Design review of the part built by this model. Coordinates are the model's own, in mm. A direction names the side the tool comes from. Coordinates: 2 decimals unless noted, no trailing zeros. Order: outer loops, then holes, each group sorted by start corner. A loop starts at its lowest first (then second) coordinate and runs counter-clockwise, first axis right, second up. Notation, with made-up numbers: M -6.75,2 L 52.25,2 A22 cw 52.25,37 Z; hole C -22,-11 d2. An arc over 180 degrees is marked long. Answer in a Markdown table with one row per item.
from build123d import *

# Parameters (mm, degrees)
SCHIZZO1_R                           = 6.5
SCHIZZO1_R_2                         = 2
BASE_FLANGIA1_DEPTH                  = 4
PIEGATURA_START                      = -26
PIEGATURA_DELLO_SCHIZZO1_OUTLINE_W   = 50
PIEGATURA_DELLO_SCHIZZO1_OUTLINE_H   = 4
PIEGATURA_DELLO_SCHIZZO1_DEPTH       = 52
PIEGATURA_START_2                    = -30
PIEGATURA_DELLO_SCHIZZO1_2_OUTLINE_R = 6.5
PIEGATURA_DELLO_SCHIZZO1_2_DEPTH     = 4
PIEGATURA_DELLO_SCHIZZO1_3_DEPTH     = 52
PIEGATURA_START_3                    = -25
PIEGATURA_DELLO_SCHIZZO1_4_DEPTH     = 50
ESTRUSIONE_ESTRUSIONE1_DEPTH         = 2


with BuildPart() as part:
    # Base-Flangia1: sheet metal written as solids
    # Schizzo1 → Base-Flangia1 (new body)
    with BuildSketch(Plane.XY):
        with BuildLine():
            Line((-25, -72), (-25, 0))
            ThreePointArc((-25, 0), (0, 25), (25, 0))
            Line((25, 0), (25, -72))
            ThreePointArc((25, -72), (23.535533906, -75.535533906), (20, -77))
            Line((20, -77), (-20, -77))
            ThreePointArc((-20, -77), (-23.535533906, -75.535533906), (-25, -72))
        make_face()
        Circle(SCHIZZO1_R, mode=Mode.SUBTRACT)
        with Locations((-12.5, -67)):
            Circle(SCHIZZO1_R_2, mode=Mode.SUBTRACT)
        with Locations((12.5, -67)):
            Circle(SCHIZZO1_R_2, mode=Mode.SUBTRACT)
    extrude(amount=-BASE_FLANGIA1_DEPTH)

    # Piegatura dello schizzo1: read off the stored shape, not the designer's step
    # Piegatura dello schizzo1 outline → Piegatura dello schizzo1 (cut)
    with BuildSketch(Plane(origin=(0, 0, 0), x_dir=(1, 0, 0), z_dir=(0, 1, 0)).offset(PIEGATURA_START)):
        with Locations((0, 2)):
            Rectangle(PIEGATURA_DELLO_SCHIZZO1_OUTLINE_W, PIEGATURA_DELLO_SCHIZZO1_OUTLINE_H)
    extrude(amount=PIEGATURA_DELLO_SCHIZZO1_DEPTH, mode=Mode.SUBTRACT)

    # Piegatura dello schizzo1 2 outline → Piegatura dello schizzo1 2 (add)
    with BuildSketch(Plane(origin=(0, 0, 0), x_dir=(1, 0, 0), z_dir=(0, 1, 0)).offset(PIEGATURA_START_2)):
        with BuildLine():
            Line((-25, 0), (-25, -26.862699383))
            ThreePointArc((-25, -26.862699383), (0, -51.862699383), (25, -26.862699383))
            Line((25, -26.862699383), (25, 0))
            Line((25, 0), (-25, 0))
        make_face()
        with Locations((0, -26.862699383)):
            Circle(PIEGATURA_DELLO_SCHIZZO1_2_OUTLINE_R, mode=Mode.SUBTRACT)
    extrude(amount=PIEGATURA_DELLO_SCHIZZO1_2_DEPTH)

    # Piegatura dello schizzo1 3 outline → Piegatura dello schizzo1 3 (cut)
    with BuildSketch(Plane.YZ.offset(PIEGATURA_START)):
        with BuildLine():
            ThreePointArc((-26, 0.01), (-27.174501807, -2.825498193), (-30.01, -4))
            Line((-30.01, -4), (-26, -4))
            Line((-26, -4), (-26, 0.01))
        make_face()
    extrude(amount=PIEGATURA_DELLO_SCHIZZO1_3_DEPTH, mode=Mode.SUBTRACT)

    # Piegatura dello schizzo1 4 outline → Piegatura dello schizzo1 4 (add)
    with BuildSketch(Plane.YZ.offset(PIEGATURA_START_3)):
        with BuildLine():
            ThreePointArc((-30, 0.01), (-30.002928932, 0.002928932), (-30.01, 0))
            Line((-30.01, 0), (-30, 0))
            Line((-30, 0), (-30, 0.01))
        make_face()
    extrude(amount=PIEGATURA_DELLO_SCHIZZO1_4_DEPTH)

    # Schizzo13 → Estrusione-Estrusione1 (add)
    with BuildSketch(Plane.ZY.offset(25)):
        with BuildLine():
            Line((0.01, -30), (15, -30))
            Line((15, -30), (0, -45))
            Line((0, -45), (0, -30.01))
            ThreePointArc((0, -30.01), (0.002928932, -30.002928932), (0.01, -30))
        make_face()
    estrusione_estrusione1 = extrude(amount=-ESTRUSIONE_ESTRUSIONE1_DEPTH)

    # Specchia1: Estrusione-Estrusione1 across plane
    add(estrusione_estrusione1.mirror(Plane(origin=(0, 0, 0), x_dir=(0, 0, 1), z_dir=(1, 0, 0))))


solid = part.part
(1) Insertion check: pin 1 Ø23.5 at (x, y) = (-5.5, -54) entering from +Z; pin 2 Ø17 at (x, z) = (0, 26.86) entering from -Y. Each pin has a flat end and moves straight along its axis. Give the tip position at first contact, or say it passes through.
Return value:
| item | result |
|---|---|
| pin 1 | stops at z = 0 |
| pin 2 | stops at y = -30 |
(2) For faces 1 (the flat face through (0, -30, 20)), 2 (the flat face through (24, -37, 8)), list the 3-axis set-ups (+Z, -Z, +X, -X, +Y, -Y) from which the entire face can be reached by the end or side of a thin tool; tool diameter is ignored.
Return value:
| item | result |
|---|---|
| face 1 | +Z, -Y |
| face 2 | +Z, +X, -X, -Y |
(3) Draft analysis for pull direction Z (two halves, no side actions). For faces 3 (the flat face through (0, -77, -2)), 4 (the cylindrical face through (-0.55, -28.028, 51.857)), 5 (the cylindrical face through (-0.35, -27.14, -2.79)), 6 (the cylindrical face through (-0.85, -28.03, 20.42)), state which applies: pulls with the +Z half, pulls with the -Z half, needs draft (parallel to the pull), parting line crosses it, or undercut.
Return value:
| item | result |
|---|---|
| face 3 | needs draft |
| face 4 | pulls with the +Z half |
| face 5 | pulls with the -Z half |
| face 6 | undercut |
(4) Add section C-C, the plane z = 14. Give the boundary of the cut face in (x, y).
Return value:
| item | result |
|---|---|
| outline | M -25,-31 L -23,-31 L -23,-30 L 23,-30 L 23,-31 L 25,-31 L 25,-26 L -25,-26 Z |
(5) Add section B-B, the plane y = -68. Give the boundary of the cut face in (x, z).
Return value:
| item | result |
|---|---|
| outline | M -25,-4 L -14.23,-4 L -14.23,0 L -25,0 Z; M -10.77,-4 L 10.77,-4 L 10.77,0 L -10.77,0 Z; M 14.23,-4 L 25,-4 L 25,0 L 14.23,0 Z |
(6) For line 1 along X through (y, z) = (-34, 7.5); line 2 along Y through (x, z) = (-16, 46); line 3 along Y through (x, z) = (-12.5, -1.45), list the stretches that pass through material, from the lowest coordinate up. Write a range as from..to.
Return value:
| item | result |
|---|---|
| line 1 | x = -25..-23, 23..25 |
| line 2 | y = -30..-26 |
| line 3 | y = -77..-69, -65..-26.28 |
